from build123d import *

# Parameters (mm, degrees)
F1_DEPTH = 8


with BuildPart() as f1:
    # F0 (on Top) → F1 (new body)
    with BuildSketch(Plane.XY):
        with BuildLine():
            Line((25, 38.661759), (-25, 38.661759))
            Line((-25, 38.661759), (-25, 0))
            ThreePointArc((-25, 0), (-18.166248, -22.36068), (0, -37.080992))
            ThreePointArc((0, -37.080992), (18.166248, -22.36068), (25, 0))
            Line((25, 0), (25, 38.661759))
        make_face()
    extrude(amount=F1_DEPTH)


solid = f1.part
Source: CAD feature listing. Evaluate the final solid. Frame: model axes, mm. Coordinates: 2 decimals unless noted, no trailing zeros. Order: outer loops, then holes, each group sorted by start corner. A loop starts at its lowest first (then second) coordinate and runs counter-clockwise, first axis right, second up. Notation, with made-up numbers: M 35,13 L 84,13 A8 ccw 84,22 Z; hole C -16.5,-12 d1. An arc over 180 degrees is marked long. Write each question's results on one line, items separated by ' | '. Start each with the question number.
Item 1: Cut plane B-B (x = -17). Return loops of the section in (y, z).
Item 2: Cut plane A-A (z = 3.25). Return loops of the section in (x, y), and give its area (3 significant figures).
Item 3: Line query: probe 1 along X at (y, z) = (-1, 1); probe 2 along Y at (x, z) = (12, 4); probe 3 along Y at (x, z) = (-10, 2). Output: solid intervals per line, ascending.
Item 4: First-contact query: pin 1 Ø1.5 at (x, z) = (7, 3) entering from -Y; pin 2 Ø3 at (x, z) = (14.5, 2.5) entering from -Y. Flat tips, straight axial feed; report the tip coordinate or a pass-through.
Item 5: Cut plane C-C (y = -24.5). Return loops of the section in (x, z).
Checked values:
1) outline: M -24,0 L 38.66,0 L 38.66,8 L -24,8 Z
2) outline: M -25,0 A40 ccw 0,-37.08 A40 ccw 25,0 L 25,38.66 L -25,38.66 Z | area: 3,280 mm2
3) probe 1: x = -24.99 to 24.99 | probe 2: y = -29.51 to 38.66 | probe 3: y = -31.22 to 38.66
4) pin 1: stops at y = -33.89 | pin 2: stops at y = -28.57
5) outline: M -16.62,0 L 16.62,0 L 16.62,8 L -16.62,8 Z
